Verification items for the finished model (mm, model axes). Give positions to 0.01 mm unless a question says otherwise; leave off trailing zeros. Write each loop counter-clockwise with the first axis right and the second up, starting at its lowest first coordinate (ties: lowest second). Pieces come first, ordered by that corner, then holes.
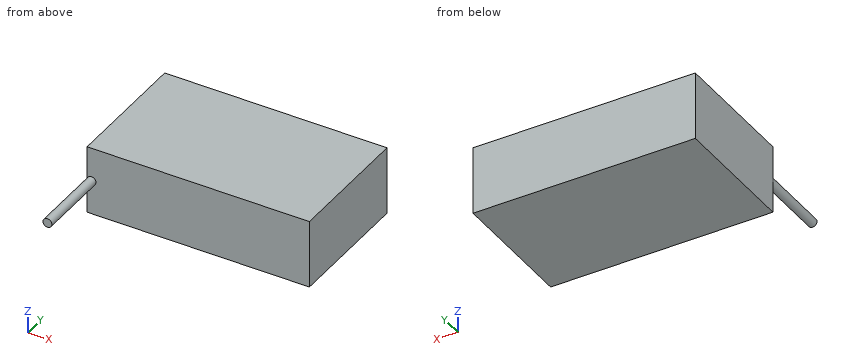
from build123d import *

# Parameters (mm, degrees)
F1_DEPTH = 23
F3_DEPTH = 25


# Not quite as in the source:
# - the program builds the solid bodies; features that only make, move or delete a surface that nothing else refers to are left out


with BuildPart() as f1:
    # F0 (on Top) → F1 (new body)
    with BuildSketch(Plane.XY):
        Polygon((-37.5, 22), (-37.5, -22), (-15.1, -22), (37.5, -22), (37.5, 22), (-15.1, 22), align=None)
    extrude(amount=F1_DEPTH)

    # F2 (on face) → F3 (join)
    with BuildSketch(Plane.XZ.offset(22)):
        with BuildLine():
            ThreePointArc((-37.5, 11.5), (-36, 10), (-34.5, 11.5))
            ThreePointArc((-34.5, 11.5), (-36, 13), (-37.5, 11.5))
        make_face()
    extrude(amount=F3_DEPTH)


solid = f1.part
Item 1: Sectioned sample at C-C on y = -35.5. Record the cut outline in (x, z), then the cut area to 3 significant figures.
Answer key:
outline: circle Ø3 at (-36, 11.5)
area: 7.07 mm2
Item 2: Sectioned sample at D-D on x = -11. Record the cut outline in (y, z).
Answer key:
outline: (-22, 0) - (22, 0) - (22, 23) - (-22, 23) - close
Item 3: Sectioned sample at B-B on z = 16.25. Record the cut outline in (x, y), then the cut area to 3 significant figures.
Answer key:
outline: (-37.5, -22) - (37.5, -22) - (37.5, 22) - (-37.5, 22) - close
area: 3,300 mm2
Item 4: Sectioned sample at A-A on x = -36. Record the cut outline in (y, z).
Answer key:
outline: (-47, 10) - (-22, 10) - (-22, 0) - (22, 0) - (22, 23) - (-22, 23) - (-22, 13) - (-47, 13) - close
Item 5: Depth check by flat-ended pin: pin 1 (4 mm diameter, centred on y = -39.5, z = 11, fed in from +X). Enter the tip coordinate at first touch or a pass-through.
Answer key:
pin 1: stops at x = -34.5
Item 6: Scan lines: line 1 along X through (y, z) = (-24, 11.75); line 2 along Y through (x, z) = (19, 8). Record each from-to range of solid material in increasing order.
Answer key:
line 1: x = -37.48 to -34.52
line 2: y = -22 to 22
